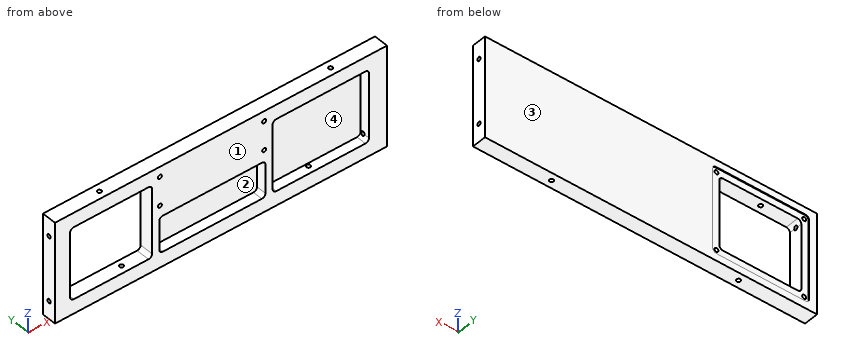
from build123d import *

# Parameters (mm, degrees)
SKETCH1_W           = 461.60558249
SKETCH1_H           = 20
BOSS_EXTRUDE1_DEPTH = 140
SKETCH2_W           = 150
SKETCH2_H           = 12
CUT_EXTRUDE1_DEPTH  = 80
CUT_EXTRUDE2_DEPTH  = 271.684185808
CUT_EXTRUDE3_DEPTH  = 1
SKETCH5_R           = 2.75
CUT_EXTRUDE4_DEPTH  = 12
FILLET1_R           = 5
SKETCH7_R           = 2.75
CUT_EXTRUDE6_DEPTH  = 30
SKETCH8_R           = 2.75
CUT_EXTRUDE7_DEPTH  = 30
BOSS_EXTRUDE2_DEPTH = 12
SKETCH10_R          = 2.75
CUT_EXTRUDE8_DEPTH  = 12
CUT_EXTRUDE5_DEPTH  = 14
SKETCH11_R          = 2.75
CUT_EXTRUDE9_DEPTH  = 30


with BuildPart() as part:
    # Sketch1 → Boss-Extrude1 (new body)
    with BuildSketch(Plane.XY):
        with Locations((0, 417)):
            Rectangle(SKETCH1_W, SKETCH1_H)
    extrude(amount=BOSS_EXTRUDE1_DEPTH)

    # Sketch2 → Cut-Extrude1 (cut)
    with BuildSketch(Plane.XY.offset(140)):
        with Locations((19.197208755, 413)):
            Rectangle(SKETCH2_W, SKETCH2_H)
    extrude(amount=-CUT_EXTRUDE1_DEPTH, mode=Mode.SUBTRACT)

    # Sketch3 → Cut-Extrude2 (cut, through all)
    with BuildSketch(Plane.XZ.offset(-407)):
        with BuildLine():
            Line((-100.802791245, 20), (-204.802791245, 20))
            ThreePointArc((-204.802791245, 20), (-208.338325151, 21.464466094), (-209.802791245, 25))
            Line((-209.802791245, 25), (-209.802791245, 115))
            ThreePointArc((-209.802791245, 115), (-208.338325151, 118.535533906), (-204.802791245, 120))
            Line((-204.802791245, 120), (-100.802791245, 120))
            ThreePointArc((-100.802791245, 120), (-97.267257339, 118.535533906), (-95.802791245, 115))
            Line((-95.802791245, 115), (-95.802791245, 25))
            ThreePointArc((-95.802791245, 25), (-97.267257339, 21.464466094), (-100.802791245, 20))
        make_face()
    extrude(amount=-CUT_EXTRUDE2_DEPTH, mode=Mode.SUBTRACT)

    # Sketch4 → Cut-Extrude3 (cut)
    with BuildSketch(Plane(origin=(0, 427, 0), x_dir=(1, 0, 0), z_dir=(0, 1, 0))):
        with BuildLine():
            Line((-90.802791245, -130), (-214.802791245, -130))
            ThreePointArc((-214.802791245, -130), (-218.338325151, -128.535533906), (-219.802791245, -125))
            Line((-219.802791245, -125), (-219.802791245, -15))
            ThreePointArc((-219.802791245, -15), (-218.338325151, -11.464466094), (-214.802791245, -10))
            Line((-214.802791245, -10), (-90.802791245, -10))
            ThreePointArc((-90.802791245, -10), (-87.267257339, -11.464466094), (-85.802791245, -15))
            Line((-85.802791245, -15), (-85.802791245, -125))
            ThreePointArc((-85.802791245, -125), (-87.267257339, -128.535533906), (-90.802791245, -130))
        make_face()
    extrude(amount=-CUT_EXTRUDE3_DEPTH, mode=Mode.SUBTRACT)

    # Sketch5 → Cut-Extrude4 (cut)
    with BuildSketch(Plane(origin=(0, 426, 0), x_dir=(1, 0, 0), z_dir=(0, 1, 0))):
        with Locations(Location((-91.802791245, -124, 0), (0, 0, 270))):
            Circle(SKETCH5_R)
        with Locations(Location((-213.802791245, -124, 0), (0, 0, 90))):
            Circle(SKETCH5_R)
        with Locations(Location((-213.802791245, -16, 0), (0, 0, 270))):
            Circle(SKETCH5_R)
        with Locations(Location((-91.802791245, -16, 0), (0, 0, 90))):
            Circle(SKETCH5_R)
    extrude(amount=-CUT_EXTRUDE4_DEPTH, mode=Mode.SUBTRACT)

    # Fillet1
    fillet1_edges = [part.edges().sort_by_distance(p)[0] for p in [
        (94.197208755, 413, 60),
        (-55.802791245, 413, 60),
    ]]
    fillet(fillet1_edges, radius=FILLET1_R)

    # Sketch7 → Cut-Extrude6 (cut)
    with BuildSketch(Plane.ZY.offset(230.802791245)):
        with Locations((25, 417)):
            Circle(SKETCH7_R)
        with Locations(Location((115, 417, 0), (0, 0, 270))):
            Circle(SKETCH7_R)
    cut_extrude6 = extrude(amount=-CUT_EXTRUDE6_DEPTH, mode=Mode.SUBTRACT)

    # Mirror1: Cut-Extrude6 across plane
    add(cut_extrude6.mirror(Plane(origin=(0, 0, 0), x_dir=(0, 0, 1), z_dir=(1, 0, 0))), mode=Mode.SUBTRACT)

    # Sketch8 → Cut-Extrude7 (cut)
    with BuildSketch(Plane.XY.offset(140)):
        with Locations((-160.802791245, 417)):
            Circle(SKETCH8_R)
        with Locations(Location((160.802791245, 417, 0), (0, 0, 180))):
            Circle(SKETCH8_R)
    extrude(amount=-CUT_EXTRUDE7_DEPTH, mode=Mode.SUBTRACT)

    # Sketch9 → Boss-Extrude2 (add)
    with BuildSketch(Plane.XZ.offset(-419)):
        with BuildLine():
            Line((94.197208755, 65), (94.197208755, 140))
            Line((94.197208755, 140), (-55.802791245, 140))
            Line((-55.802791245, 140), (-55.802791245, 65))
            ThreePointArc((-55.802791245, 65), (-54.338325151, 61.464466094), (-50.802791245, 60))
            Line((-50.802791245, 60), (89.197208755, 60))
            ThreePointArc((89.197208755, 60), (92.732742661, 61.464466094), (94.197208755, 65))
        make_face()
    extrude(amount=BOSS_EXTRUDE2_DEPTH)

    # Sketch10 → Cut-Extrude8 (cut)
    with BuildSketch(Plane.XZ.offset(-407)):
        with Locations(Location((-85, 126, 0), (0, 0, 270))):
            Circle(SKETCH10_R)
        with Locations(Location((-85, 86, 0), (0, 0, 270))):
            Circle(SKETCH10_R)
        with Locations(Location((60, 126, 0), (0, 0, 270))):
            Circle(SKETCH10_R)
        with Locations(Location((60, 86, 0), (0, 0, 270))):
            Circle(SKETCH10_R)
    extrude(amount=-CUT_EXTRUDE8_DEPTH, mode=Mode.SUBTRACT)

    # Sketch6 → Cut-Extrude5 (cut)
    with BuildSketch(Plane.XZ.offset(-407)):
        with BuildLine():
            Line((200.802791245, 120), (76.802791245, 120))
            ThreePointArc((76.802791245, 120), (73.267257339, 118.535533906), (71.802791245, 115))
            Line((71.802791245, 115), (71.802791245, 25))
            ThreePointArc((71.802791245, 25), (73.267257339, 21.464466094), (76.802791245, 20))
            Line((76.802791245, 20), (200.802791245, 20))
            ThreePointArc((200.802791245, 20), (204.338325151, 21.464466094), (205.802791245, 25))
            Line((205.802791245, 25), (205.802791245, 115))
            ThreePointArc((205.802791245, 115), (204.338325151, 118.535533906), (200.802791245, 120))
        make_face()
        with BuildLine():
            Line((56.802791245, 70), (-80.802791245, 70))
            ThreePointArc((-80.802791245, 70), (-84.338325151, 68.535533906), (-85.802791245, 65))
            Line((-85.802791245, 65), (-85.802791245, 25))
            ThreePointArc((-85.802791245, 25), (-84.338325151, 21.464466094), (-80.802791245, 20))
            Line((-80.802791245, 20), (56.802791245, 20))
            ThreePointArc((56.802791245, 20), (60.338325151, 21.464466094), (61.802791245, 25))
            Line((61.802791245, 25), (61.802791245, 65))
            ThreePointArc((61.802791245, 65), (60.338325151, 68.535533906), (56.802791245, 70))
        make_face()
    extrude(amount=-CUT_EXTRUDE5_DEPTH, mode=Mode.SUBTRACT)

    # Sketch11 → Cut-Extrude9 (cut)
    with BuildSketch(Plane(origin=(0, 0, 0), x_dir=(-1, 0, 0), z_dir=(0, 0, -1))):
        with Locations((130, 417)):
            Circle(SKETCH11_R)
        with Locations((-130, 417)):
            Circle(SKETCH11_R)
    extrude(amount=-CUT_EXTRUDE9_DEPTH, mode=Mode.SUBTRACT)


solid = part.part
CAD build for the part. Positions are in the model's coordinates, mm. Face numbers are marked on the shaded views. A direction names the side the tool comes from. Give positions to 0.01 mm unless a question says otherwise; leave off trailing zeros. Loops run counter-clockwise (first coordinate to the right, second up) from the corner with the lowest first, then second, coordinate; pieces in that order, holes last. Notation, with made-up numbers: M -33.5,89 L -26.5,89 A30 ccw -26.5,113 Z; hole C 36.25,9.5 d8. An arc over 180 degrees is marked long. Answer in a Markdown table with one row per item. Add a question column.
Item 1: Band-saw the part on B-B on x = -137. Give the cut face in (y, z).
Item 2: Probe probe 1 along X at (y, z) = (416.75, 86); probe 2 along X at (y, z) = (414.75, 108); probe 3 along Z at (x, y) = (-221.75, 417). List the from-to ranges inside material, lowest first.
Item 3: Mould opens along Z. For the marked faces 3 and 4 say: +Z half, -Z half, draft (parallel to the pull), parting line (faces both ways), or undercut.
Item 4: Drop flat-ended pins along their axis: P1, Ø4, axis at x = -4.5, y = 410.5, coming from the -Z side; P2, Ø1.6, axis at x = -213, z = 125, coming from the +Y side; P3, Ø1.6, axis at x = 61, z = 86.5, coming from the -Y side; P4, Ø8, axis at x = 143.5, z = 36, coming from the -Y side. Give the stop position or say it passes through.
Item 5: Band-saw the part on A-A on y = 410.75. Give the number of separate pieces and of enclosed holes in the cut face, then the cut area to 3 significant figures.
Item 6: Tool access for the marked faces 1 and 2: list every direction of +Z, -Z, +X, -X, +Y, -Y with a clear straight run to the whole face (end or side of a thin tool).
Item 7: Band-saw the part on C-C on x = -34. Give the cut face in (y, z).
Reply:
| question | item | result |
|---|---|---|
| 1 | outline | M 407,0 L 427,0 L 427,10 L 426,10 L 426,20 L 407,20 Z; M 407,120 L 426,120 L 426,130 L 427,130 L 427,140 L 407,140 Z |
| 2 | probe 1 | x = -230.8 to -209.8, -95.8 to -87.75, -82.25 to 57.25, 62.75 to 71.8, 205.8 to 230.8 |
| 2 | probe 2 | x = -230.8 to -209.8, -95.8 to 71.8, 205.8 to 230.8 |
| 2 | probe 3 | z = 0 to 22.25, 27.75 to 112.25, 117.75 to 140 |
| 3 | face 3 | draft |
| 3 | face 4 | undercut |
| 4 | P1 | stops at z = 0 |
| 4 | P2 | stops at y = 414 |
| 4 | P3 | stops at y = 419 |
| 4 | P4 | stops at y = 421 |
| 5 | separate pieces | 1 |
| 5 | enclosed holes | 7 |
| 5 | area | 32,400 mm^2 |
| 6 | face 1 | +Z, -Z, +X, -X, -Y |
| 6 | face 2 | -Y |
| 7 | outline | M 407,0 L 427,0 L 427,140 L 407,140 L 407,70 L 421,70 L 421,20 L 407,20 Z |
